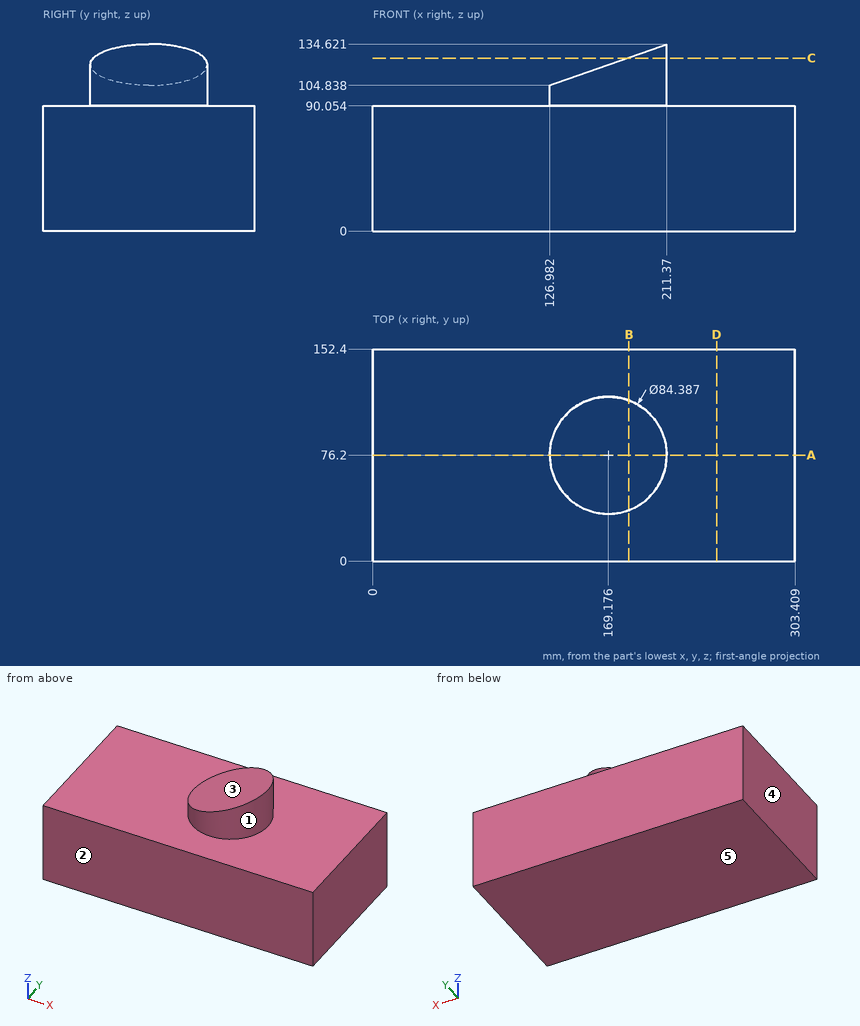
Design review of the part shown in the three views and the two pictorial views. Dimensions are in mm from the part's minimum x, y and z. A direction names the side the tool comes from. Give positions to 0.01 mm unless a question says otherwise; leave off trailing zeros. Loops run counter-clockwise (first coordinate to the right, second up) from the corner with the lowest first, then second, coordinate; pieces in that order, holes last. Notation, with made-up numbers: (26.5, -31) - (75.5, -31) arc R28 ccw to (75.5, 5) - close; hole circle Ø6 at (-33.5, -13). An arc over 180 degrees is marked (long way). Answer as a JSON object with one key per item and string values.
Q1. Add section C-C on z = 124.5. State the section outline as (x, y) points, plus the area to 3 significant figures.
Worked out:
{"outline": "(182.69, 36.23) arc R42.19 ccw to (182.69, 116.17) - close", "area": "1,680 mm^2"}
Q2. Add section B-B on x = 184. State the section outline as (y, z) points (1 decimal), plus the area to 3 significant figures.
Worked out:
{"outline": "(0, 0) - (152.4, 0) - (152.4, 90.1) - (115.7, 90.1) - (115.7, 125) - (36.7, 125) - (36.7, 90.1) - (0, 90.1) - close", "area": "16,500 mm^2"}
Q3. Add section A-A on y = 76.2. State the section outline as (x, z) points (1 decimal).
Worked out:
{"outline": "(0, 0) - (303.4, 0) - (303.4, 90.1) - (211.4, 90.1) - (211.4, 134.6) - (127, 104.8) - (127, 90.1) - (0, 90.1) - close"}
Q4. Mouldability with a two-part tool opening along Z and no side actions: class the marked faces 3, 4 and 5 as +Z half, -Z half, draft (parallel to the pull), parting line (faces both ways), or undercut.
Worked out:
{"face 3": "+Z half", "face 4": "draft", "face 5": "-Z half"}
Q5. Insertion check: pin 1 (2 mm diameter, centred on y = 53, z = 108, fed in from -X); pin 2 (6 mm diameter, centred on x = 170, y = 103, fed in from +Z); pin 3 (1 mm diameter, centred on x = 252, y = 63, fed in from +Z). Each pin has a flat end and moves straight along its axis. Give the tip position at first contact, or say it passes through.
Worked out:
{"pin 1": "stops at x = 133.58", "pin 2": "stops at z = 121.08", "pin 3": "stops at z = 90.05"}
Q6. To check wall thickness, follow line 1 along Z through (x, y) = (38.5, 92.5) (1 decimal); line 2 along X through (y, z) = (107, 99) (1 decimal); line 3 along Z through (x, y) = (135, 85). State the ranges of each line that lie inside material, in increasing order.
Worked out:
{"line 1": "z = 0 to 90.1", "line 2": "x = 140.3 to 198", "line 3": "z = 0 to 107.67"}
Q7. Add section D-D on x = 247. State the section outline as (y, z) points (1 decimal), plus the area to 3 significant figures.
Worked out:
{"outline": "(0, 0) - (152.4, 0) - (152.4, 90.1) - (0, 90.1) - close", "area": "13,700 mm^2"}
Q8. For the marked faces 1 and 2, list the 3-axis set-ups (+Z, -Z, +X, -X, +Y, -Y) from which the entire face can be reached by the end or side of a thin tool; tool diameter is ignored.
Worked out:
{"face 1": "+Z", "face 2": "+Z, -Z, +X, -X, -Y"}
